from build123d import *

# Parameters (mm, degrees)
SKETCH2_R          = 2
CUT_EXTRUDE1_DEPTH = 11.862780491


with BuildPart() as part:
    # Sketch1 → Revolve1 (revolve)
    with BuildSketch(Plane.XY, mode=Mode.PRIVATE) as revolve1_sk:
        Polygon((0, 0), (0, 5), (-3, 5), (-3, 2.5), (-2.5, 2.5), (-2.5, 0), align=None)
    revolve1 = revolve(revolve1_sk.sketch.rotate(Axis((0, 0, 0), (0, 1, 0)), 270), axis=Axis((0, 0, 0), (0, 1, 0)))

    # Mirror1: Revolve1 across plane
    add(revolve1.mirror(Plane(origin=(-2.5, 0, 0), x_dir=(0, 0, 1), z_dir=(0, 1, 0))))

    # Sketch2 → Cut-Extrude1 (cut, through all)
    with BuildSketch(Plane(origin=(0, 5, 0), x_dir=(1, 0, 0), z_dir=(0, 1, 0))):
        with Locations(Location((0, 0, 0), (0, 0, 270))):
            Circle(SKETCH2_R)
    extrude(amount=-CUT_EXTRUDE1_DEPTH, mode=Mode.SUBTRACT)


solid = part.part
Read the model definition and answer for the solid it produces. Units are mm, in the model's axes. A direction names the side the tool comes from. Coordinates: 2 decimals unless noted, no trailing zeros. Write each loop counter-clockwise with the first axis right and the second up, starting at its lowest first coordinate (ties: lowest second). Pieces come first, ordered by that corner, then holes. Notation, with made-up numbers: (60.5, -35.5) - (110.5, -35.5) arc R12 cw to (110.5, -14.5) - close; hole circle Ø4 at (13.5, 77.25). An arc over 180 degrees is marked (long way). One line per question, with ' | ' between items.
Q1. For faces 1 (the cylindrical face through (-2, 0, 0)), 2 (the flat face through (-2, 2.5, 2)), determine the directions among +Z, -Z, +X, -X, +Y, -Y from which every point of the face is accessible in a straight line to the end or side of a thin tool.
Result set:
face 1: +Y, -Y | face 2: none
Q2. Find section B-B, the plane x = 0. Write down the section's boundary in (y, z).
Result set:
outline: (-5, -3) - (-2.5, -3) - (-2.5, -2.5) - (2.5, -2.5) - (2.5, -3) - (5, -3) - (5, -2) - (-5, -2) - close; (-5, 2) - (5, 2) - (5, 3) - (2.5, 3) - (2.5, 2.5) - (-2.5, 2.5) - (-2.5, 3) - (-5, 3) - close
Q3. Consider L1, parallel to Y at x = 2, z = -2; L2, parallel to X at y = 4.25, z = -1.6; L3, parallel to X at y = 3, z = 1.35. Determine where each line is inside the solid, lowest interval first. Write a range as [from, to].
Result set:
L1: [-5, -2.5], [2.5, 5] | L2: [-2.54, -1.2], [1.2, 2.54] | L3: [-2.68, -1.48], [1.48, 2.68]
Q4. Each of these flat-tipped pins is pushed along its axis until it touches: P1, Ø1, axis at x = -1, y = -0.5, coming from the +Z side; P2, Ø3, axis at x = 0.5, z = 1.5, coming from the +Y side; P3, Ø1.5, axis at x = 1.5, y = -2.5, coming from the -Z side; P4, Ø1, axis at x = -1.5, y = -2.5, coming from the -Z side. Where does it stop, or does it pass through?
Result set:
P1: z = 2.45 | P2: y = 5 | P3: z = -2.9 | P4: z = -2.83
Q5. Find section A-A, the plane z = 0. Write down the section's boundary in (x, y), plus the area to 3 significant figures.
Result set:
outline: (-3, -5) - (-2, -5) - (-2, 5) - (-3, 5) - (-3, 2.5) - (-2.5, 2.5) - (-2.5, -2.5) - (-3, -2.5) - close; (2, -5) - (3, -5) - (3, -2.5) - (2.5, -2.5) - (2.5, 2.5) - (3, 2.5) - (3, 5) - (2, 5) - close | area: 15.0 mm^2
Q6. Find section C-C, the plane y = 4.5. Write down the section's boundary in (x, z), plus the area to 3 significant figures.
Result set:
outline: circle Ø6 at (0, 0); hole circle Ø4 at (0, 0) | area: 15.7 mm^2
Q7. Determine the mould class of faces 3 (the flat face through (2, -5, 1)), 4 (the flat face through (-2, -2.5, 2)), 5 (the flat face through (2, 5, 1)) for opening direction Y: +Y half, -Y half, draft (parallel to the pull), parting line (faces both ways), or undercut.
Result set:
face 3: -Y half | face 4: undercut | face 5: +Y half
Q8. Find section D-D, the plane x = -2.25. Write down the section's boundary in (y, z), plus the area to 3 significant figures.
Result set:
outline: (-5, -1.98) - (-2.5, -1.98) - (-2.5, -1.09) - (2.5, -1.09) - (2.5, -1.98) - (5, -1.98) - (5, 1.98) - (2.5, 1.98) - (2.5, 1.09) - (-2.5, 1.09) - (-2.5, 1.98) - (-5, 1.98) - close | area: 30.7 mm^2
